Drawing for the job (mm, zero at the part's lowest x, y, z). Give positions to 0.01 mm unless a question says otherwise; leave off trailing zeros. Write each loop counter-clockwise with the first axis right and the second up, starting at its lowest first coordinate (ties: lowest second). Pieces come first, ordered by that corner, then holes.
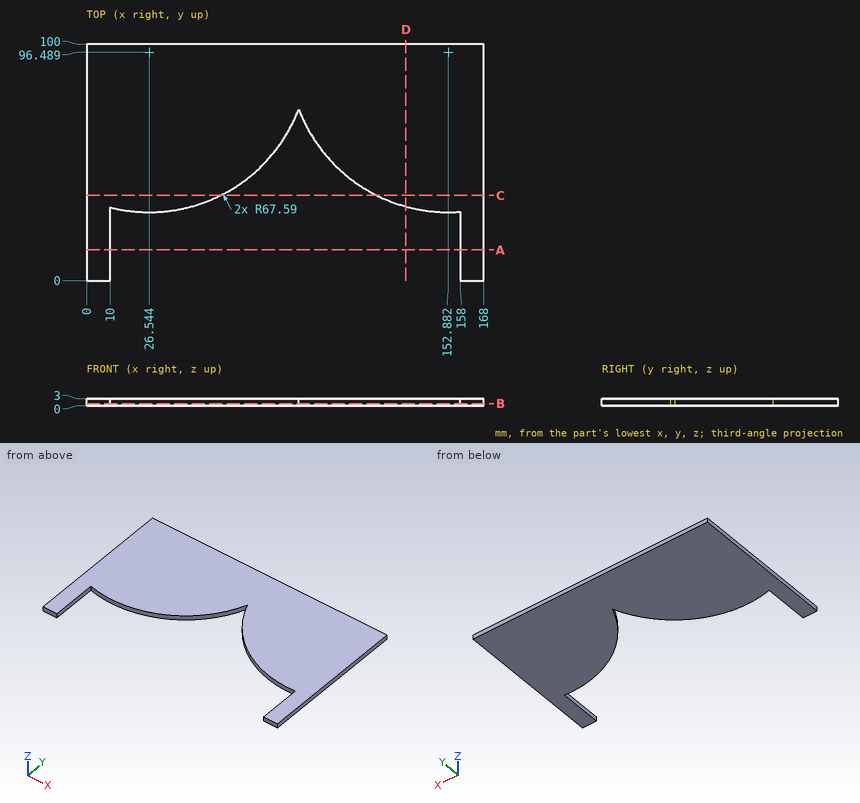
1. Slice it at A-A, the plane y = 13. Write the cut outline in (x, z).
Calculated:
outline: (0, 0) - (10, 0) - (10, 3) - (0, 3) - close; (158, 0) - (168, 0) - (168, 3) - (158, 3) - close
2. Slice it at C-C, the plane y = 36. Write the cut outline in (x, z), and give its area (3 significant figures).
Calculated:
outline: (0, 0) - (56.7, 0) - (56.7, 3) - (0, 3) - close; (122.72, 0) - (168, 0) - (168, 3) - (122.72, 3) - close
area: 306 mm2
3. Slice it at B-B, the plane z = 0.9. Write the cut outline in (x, y) (1 decimal), and give its area (3 significant figures).
Calculated:
outline: (0, 0) - (10, 0) - (10, 31) arc R67.6 ccw to (89.7, 72.4) arc R67.6 ccw to (158, 29.1) - (158, 0) - (168, 0) - (168, 100) - (0, 100) - close
area: 11,000 mm2
4. Probe probe 1 along X at (y, z) = (27.5, 2.15); probe 2 along Y at (x, z) = (26, 0.45); probe 3 along X at (y, z) = (47, 2.9) (1 decimal). List the from-to ranges inside material, lowest first.
Calculated:
probe 1: x = 0 to 10, 158 to 168
probe 2: y = 28.9 to 100
probe 3: x = 0 to 72.6, 106.8 to 168
5. Slice it at D-D, the plane x = 135. Write the cut outline in (y, z).
Calculated:
outline: (31.31, 0) - (100, 0) - (100, 3) - (31.31, 3) - close
